Part model, mm, in its own coordinate system. A direction names the side the tool comes from. Give positions to 0.01 mm unless a question says otherwise; leave off trailing zeros. Order: outer loops, then holes, each group sorted by start corner. A loop starts at its lowest first (then second) coordinate and runs counter-clockwise, first axis right, second up. Notation, with made-up numbers: (70, 73.5) - (99, 73.5) arc R12 ccw to (99, 91.5) - close; hole circle Ø8 at (50.5, 38.25). An arc over 180 degrees is marked (long way). Use one line per item in the form item = value. Start each with the question number.
1. Pull direction Z, two halves, no side cores. Call faces 1 (the face through (-135.25, 3, -4)), 2 (the face through (128.105, 2.662, -79.615)), 3 (the face through (-12.659, 2.662, -86.733)), 4 (the face through (-2, 3, -95)): +Z half, -Z half, draft (parallel to the pull), parting line (faces both ways), or undercut.
2. Band-saw the part on C-C, the plane x = 25. List the corners of the cut face in (y, z).
3. Pin check, flat tip, straight feed: P1, Ø4, axis at x = 14, z = -83.5, coming from the -Y side. Stop position of the tip, or through.
4. Band-saw the part on A-A, the plane x = -14. List the corners of the cut face in (y, z).
5. Drill centre lines: line 1 (X direction, y = 4, z = -10); line 2 (X direction, y = 3.7, z = -83.5); line 3 (X direction, y = 2.4, z = -38). Where is each one in solid material? Low to high.
6. Tool access for faces 5 (the face through (-35, 3.2, -67)), 6 (the face through (-2, 5.4, -66)): list every direction of +Z, -Z, +X, -X, +Y, -Y with a clear straight run to the whole face (end or side of a thin tool).
7. Band-saw the part on B-B, the plane z = -16. List the corners of the cut face in (x, y), plus the area to 3 significant figures.
from build123d import *

# Parameters (mm, degrees)
SKETCH1_W           = 270.5
SKETCH1_H           = 180
SKETCH1_R           = 2
SKETCH1_R_2         = 3.5
SKETCH1_W_2         = 222.5
SKETCH1_H_2         = 136
BOSS_EXTRUDE1_DEPTH = 5.4
SKETCH1_5_W         = 230.5
SKETCH1_5_H         = 150
CUT_EXTRUDE1_DEPTH  = 3.2


with BuildPart() as part:
    # Sketch1 → Boss-Extrude1 (new body)
    with BuildSketch(Plane(origin=(0, 0, 0), x_dir=(1, 0, 0), z_dir=(0, 1, 0))):
        with Locations((0, 5)):
            Rectangle(SKETCH1_W, SKETCH1_H)
        with Locations(Location((-125.25, -10, 0), (0, 0, 90))):
            Circle(SKETCH1_R, mode=Mode.SUBTRACT)
        with Locations(Location((125.25, -10, 0), (0, 0, 90))):
            Circle(SKETCH1_R, mode=Mode.SUBTRACT)
        with Locations(Location((-125.25, 10, 0), (0, 0, 90))):
            Circle(SKETCH1_R, mode=Mode.SUBTRACT)
        with Locations(Location((-125, 38, 0), (0, 0, 90))):
            Circle(SKETCH1_R_2, mode=Mode.SUBTRACT)
        with Locations(Location((-125, 78, 0), (0, 0, 90))):
            Circle(SKETCH1_R_2, mode=Mode.SUBTRACT)
        with Locations(Location((-14, 83.5, 0), (0, 0, 90))):
            Circle(SKETCH1_R_2, mode=Mode.SUBTRACT)
        with Locations((0, -3)):
            Rectangle(SKETCH1_W_2, SKETCH1_H_2, mode=Mode.SUBTRACT)
        with Locations(Location((125.25, 10, 0), (0, 0, 90))):
            Circle(SKETCH1_R, mode=Mode.SUBTRACT)
        with Locations(Location((125, 38, 0), (0, 0, 90))):
            Circle(SKETCH1_R_2, mode=Mode.SUBTRACT)
        with Locations(Location((14, 83.5, 0), (0, 0, 90))):
            Circle(SKETCH1_R_2, mode=Mode.SUBTRACT)
        with Locations(Location((125, 78, 0), (0, 0, 90))):
            Circle(SKETCH1_R_2, mode=Mode.SUBTRACT)
    extrude(amount=BOSS_EXTRUDE1_DEPTH)

    # Sketch1<5> → Cut-Extrude1 (cut)
    with BuildSketch(Plane(origin=(0, 0, 0), x_dir=(1, 0, 0), z_dir=(0, 1, 0))):
        Rectangle(SKETCH1_5_W, SKETCH1_5_H)
    extrude(amount=CUT_EXTRUDE1_DEPTH, mode=Mode.SUBTRACT)


solid = part.part
From the geometry:
q1.face_1 = draft
q1.face_2 = undercut
q1.face_3 = undercut
q1.face_4 = -Z half
q2.outline = (0, -95) - (5.4, -95) - (5.4, -65) - (3.2, -65) - (3.2, -75) - (0, -75) - close; (0, 75) - (3.2, 75) - (3.2, 71) - (5.4, 71) - (5.4, 85) - (0, 85) - close
q3.P1 = through
q4.outline = (0, -95) - (5.4, -95) - (5.4, -87) - (0, -87) - close; (0, -80) - (5.4, -80) - (5.4, -65) - (3.2, -65) - (3.2, -75) - (0, -75) - close; (0, 75) - (3.2, 75) - (3.2, 71) - (5.4, 71) - (5.4, 85) - (0, 85) - close
q5.line_1 = -135.25 to -127.25, -123.25 to -111.25, 111.25 to 123.25, 127.25 to 135.25
q5.line_2 = -135.25 to -17.5, -10.5 to 10.5, 17.5 to 135.25
q5.line_3 = -135.25 to -128.5, -121.5 to -115.25, 115.25 to 121.5, 128.5 to 135.25
q6.face_5 = -Y
q6.face_6 = +Z, -Z, +X, -X, +Y
q7.outline = (-135.25, 0) - (-115.25, 0) - (-115.25, 3.2) - (-111.25, 3.2) - (-111.25, 5.4) - (-135.25, 5.4) - close; (111.25, 3.2) - (115.25, 3.2) - (115.25, 0) - (135.25, 0) - (135.25, 5.4) - (111.25, 5.4) - close
q7.area = 234 mm²
